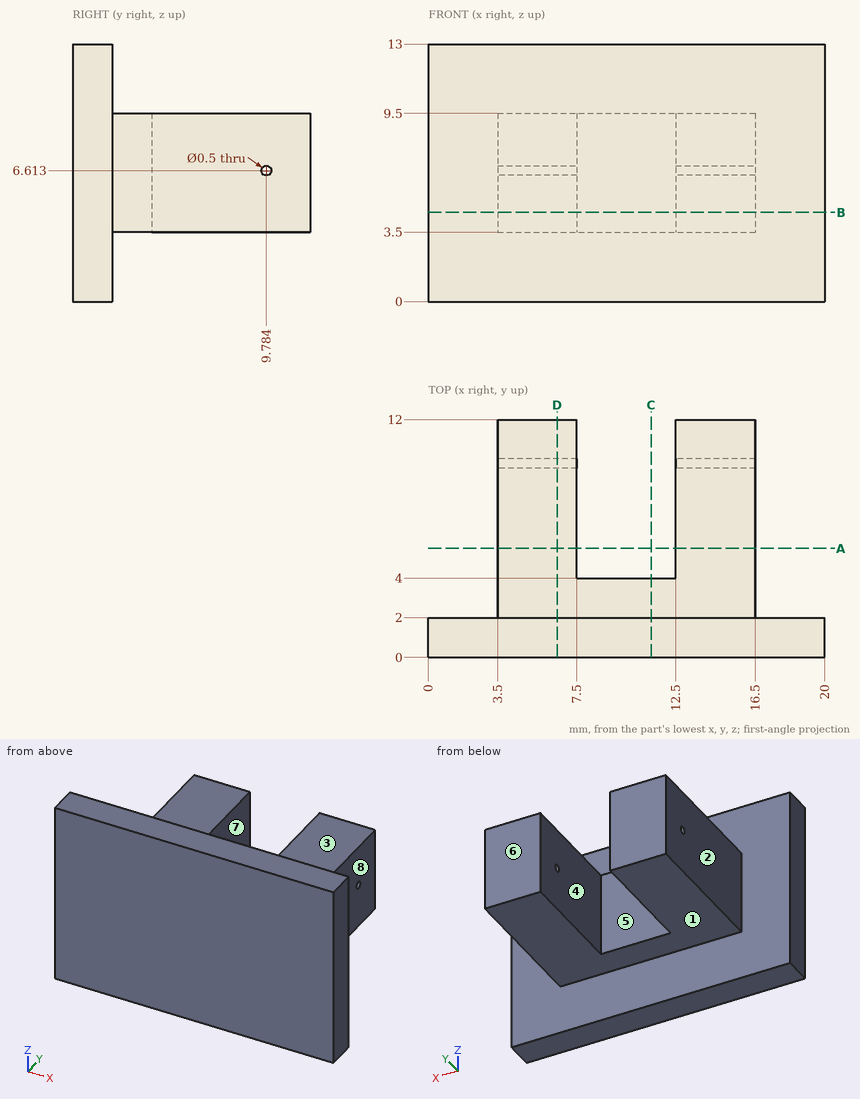
Geometry: see drawing. Coordinates: mm, zero at the bounding-box minimum. A direction names the side the tool comes from. Coordinates: 2 decimals unless noted, no trailing zeros. Write each loop counter-clockwise with the first axis right and the second up, starting at its lowest first coordinate (ties: lowest second). Pieces come first, ordered by that corner, then holes. Notation, with made-up numbers: (-14.5, 49) - (-3.5, 49) arc R28 ccw to (-3.5, 68) - close; hole circle Ø9 at (-31.5, 78). An arc over 180 degrees is marked (long way). Put each result on its own line as item: value. Start each with the question number.
1) Contact query for flat-ended pins moving along their axis: pin 1 (1.5 mm diameter, centred on x = 15.5, y = 3.5, fed in from -Z); pin 2 (6 mm diameter, centred on y = 8.5, z = 1.5, fed in from -X); pin 3 (1.8 mm diameter, centred on y = 7.5, z = 5.5, fed in from +X). Output: stop coordinate, or through.
2) Cut plane B-B (z = 4.5). Return the cut outline in (x, y).
3) Cut plane C-C (x = 11.25). Return the cut outline in (y, z).
4) Reachability of the marked faces 1, 2, 3 and 4 from +Z, -Z, +X, -X, +Y, -Y: full face, straight path, thin tool, end or side. Return the list, or none.
5) Cut plane D-D (x = 6.5). Return the cut outline in (y, z), plus the area to 3 significant figures.
6) Cut plane A-A (y = 5.5). Return the cut outline in (x, z).
7) Mould query, pull axis X, two halves, no side actions, for the marked faces 5, 6, 7 and 8. Classes: pulls with the +X half, pulls with the -X half, needs draft (parallel to the pull), parting line crosses it, or undercut.
8) Ray query, L1, parallel to X at y = 5.5, z = 6.75; L2, parallel to Y at x = 12, z = 3.25; L3, parallel to Z at x = 12.75, y = 3. Return the intervals inside material, ascending.
Resolved:
1. pin 1: stops at z = 3.5
1. pin 2: stops at x = 3.5
1. pin 3: stops at x = 16.5
2. outline: (0, 0) - (20, 0) - (20, 2) - (16.5, 2) - (16.5, 12) - (12.5, 12) - (12.5, 4) - (7.5, 4) - (7.5, 12) - (3.5, 12) - (3.5, 2) - (0, 2) - close
3. outline: (0, 0) - (2, 0) - (2, 3.5) - (4, 3.5) - (4, 9.5) - (2, 9.5) - (2, 13) - (0, 13) - close
4. face 1: -Z, +X, -X, +Y
4. face 2: +Z, -Z, -X, +Y
4. face 3: +Z, +X, -X, +Y
4. face 4: +Z, -Z, +Y
5. outline: (0, 0) - (2, 0) - (2, 3.5) - (12, 3.5) - (12, 9.5) - (2, 9.5) - (2, 13) - (0, 13) - close; hole circle Ø0.5 at (9.78, 6.61)
5. area: 85.8 mm2
6. outline: (3.5, 3.5) - (7.5, 3.5) - (7.5, 9.5) - (3.5, 9.5) - close; (12.5, 3.5) - (16.5, 3.5) - (16.5, 9.5) - (12.5, 9.5) - close
7. face 5: undercut
7. face 6: needs draft
7. face 7: undercut
7. face 8: pulls with the +X half
8. L1: x = 3.5 to 7.5, 12.5 to 16.5
8. L2: y = 0 to 2
8. L3: z = 3.5 to 9.5
